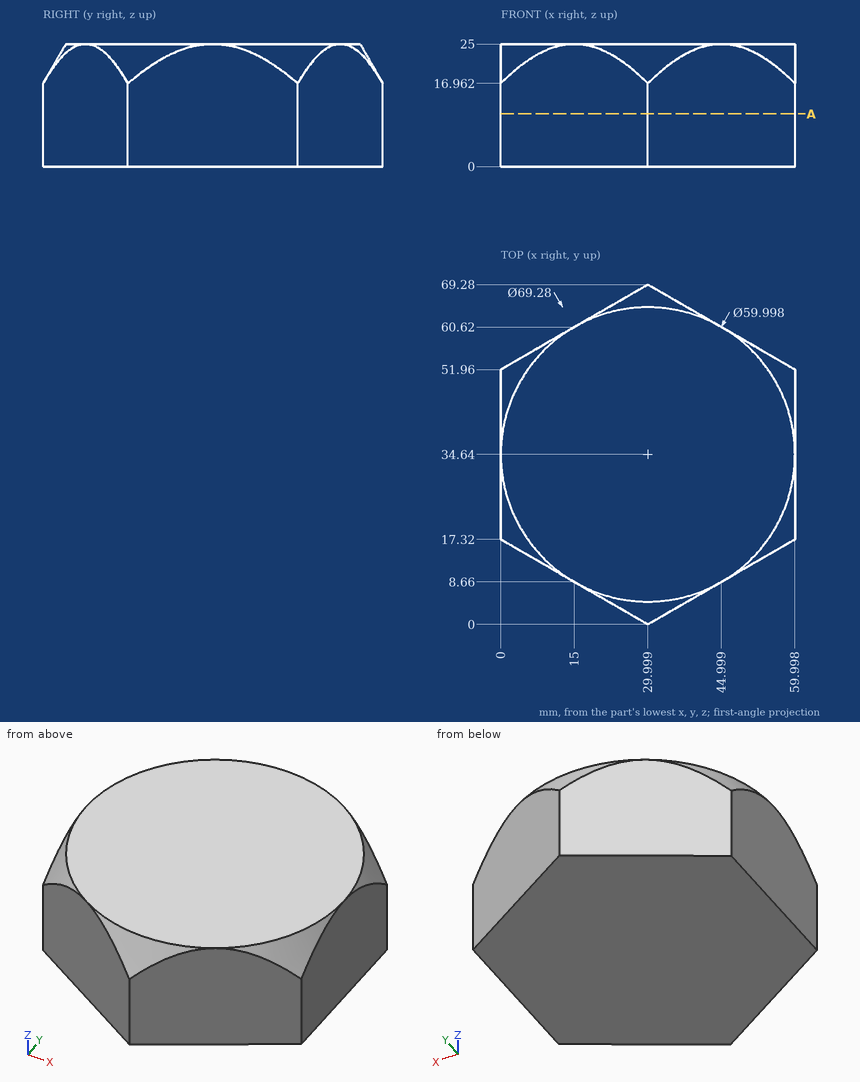
Source: three-view drawing plus pictorial views. Frame: mm from the lowest corner of the part. Round coordinates to 2 decimals unless told otherwise and drop trailing zeros. Loops run counter-clockwise (first coordinate to the right, second up) from the corner with the lowest first, then second, coordinate; pieces in that order, holes last.
1. Contact query for flat-ended pins moving along their axis: pin 1 (1.5 mm diameter, centred on x = 17, z = 20.5, fed in from +Y); pin 2 (2 mm diameter, centred on x = 48, z = 19, fed in from -Y) (1 decimal); pin 3 (5 mm diameter, centred on y = 12.5, z = 17.5, fed in from +X); pin 4 (8 mm diameter, centred on y = 53, z = 4.5, fed in from -X). Output: stop coordinate, or through.
2. Section query A-A on z = 10.75. Output: boundary loops of the cut face in (x, y).
3. Ray query, L1, parallel to Y at x = 39.5, z = 3.25 (1 decimal); L2, parallel to X at y = 49, z = 22.75; L3, parallel to X at y = 17, z = 7.25 (1 decimal). Return the intervals inside material, ascending.
Answers below:
1. pin 1: stops at y = 62.21
1. pin 2: stops at y = 9.8
1. pin 3: stops at x = 55.98
1. pin 4: stops at x = 0
2. outline: (0, 17.32) - (30, 0) - (60, 17.32) - (60, 51.96) - (30, 69.28) - (0, 51.96) - close
3. L1: y = 5.5 to 63.8
3. L2: x = 2.19 to 57.81
3. L3: x = 0.6 to 59.4
